CAD build for the part. Positions are in the model's coordinates, mm. Face numbers are marked on the shaded views. A direction names the side the tool comes from. Coordinates: 2 decimals unless noted, no trailing zeros. Loops run counter-clockwise (first coordinate to the right, second up) from the corner with the lowest first, then second, coordinate; pieces in that order, holes last. Notation, with made-up numbers: (71.5, 18.25) -> (128.5, 18.25) arc R32 cw to (128.5, 52.25) -> close; hole circle Ø8 at (50, 28). An arc over 180 degrees is marked (long way). Write item = value, one per line. Start each with the question number.
(1) Band-saw the part on A-A (z = -50). Write the cut outline in (x, y), and give its area (3 significant figures).
(2) Band-saw the part on B-B (y = 37.5). Write the cut outline in (x, z).
(3) Tool access for the marked faces 1 and 2: list every direction of +Z, -Z, +X, -X, +Y, -Y with a clear straight run to the whole face (end or side of a thin tool).
(4) Pull direction Z, two halves, no side cores. Call the marked faces 3, 4 and 5: +Z half, -Z half, draft (parallel to the pull), parting line (faces both ways), or undercut.
(5) Flat gauge pins, fed straight in: P1, Ø1.5, axis at x = 77.5, z = -70, coming from the +Y side; P2, Ø2, axis at x = 15.87, y = 58.37, coming from the +Z side; P3, Ø25, axis at x = 85, y = 65, coming from the -Z side; P4, Ø2, axis at x = 69.2, z = -73.6, coming from the +Y side. Where does each tip first touch, or does it go through?
(6) Band-saw the part on C-C (x = 59). Write the cut outline in (y, z), and give its area (3 significant figures).
(7) Drill centre lines: line 1 (Y direction, x = 30, z = -119.15); line 2 (Y direction, x = 119.15, z = -20); line 3 (Z direction, x = 58, y = 48). Where is each one in solid material? Low to high. Write a range as from..to.
(8) Band-saw the part on D-D (x = 87). Write the cut outline in (y, z), and give its area (3 significant figures).
```python
from build123d import *

# Parameters (mm, degrees)
SKETCH1_W                   = 120
SKETCH1_H                   = 120
BOSS_EXTRUDE1_DEPTH         = 90
SKETCH2_W                   = 116.2
SKETCH2_H                   = 116.2
CUT_EXTRUDE1_DEPTH          = 88
BOSS_EXTRUDE2_DEPTH         = 88
CUT_EXTRUDE2_REACH          = 194.094
SKETCH5_R                   = 4.75
SKETCH5_R_2                 = 15.75
CUT_EXTRUDE3_REACH          = 194.094
SKETCH4_R                   = 3.9
SKETCH4_R_2                 = 15.75
SKETCH4_W                   = 12
SKETCH4_H                   = 10.8
CUT_EXTRUDE4_REACH          = 194.094
SKETCH6_R                   = 4.75
SKETCH6_R_2                 = 3.4
SKETCH6_R_3                 = 9.9
M3_TAPPED_HOLE1_D           = 2.5
M3_TAPPED_HOLE1_CSINK_D     = 3.05
M3_TAPPED_HOLE1_CSINK_ANGLE = 90
M3_TAPPED_HOLE3_D           = 2.5
M3_TAPPED_HOLE3_DEPTH       = 7.5
M3_TAPPED_HOLE3_CSINK_D     = 3.05
M3_TAPPED_HOLE3_CSINK_ANGLE = 90
M3_TAPPED_HOLE3_TIP         = 0.751075774
M3_TAPPED_HOLE4_D           = 2.5
M3_TAPPED_HOLE4_DEPTH       = 7.5
M3_TAPPED_HOLE4_CSINK_D     = 3.05
M3_TAPPED_HOLE4_CSINK_ANGLE = 90
M3_TAPPED_HOLE4_TIP         = 0.751075774


with BuildPart() as part:
    # Sketch1 → Boss-Extrude1 (new body)
    with BuildSketch(Plane(origin=(0, 0, 0), x_dir=(1, 0, 0), z_dir=(0, 1, 0))):
        with Locations((60, 60)):
            Rectangle(SKETCH1_W, SKETCH1_H)
    extrude(amount=BOSS_EXTRUDE1_DEPTH)

    # Sketch2 → Cut-Extrude1 (cut)
    with BuildSketch(Plane(origin=(0, 90, 0), x_dir=(1, 0, 0), z_dir=(0, 1, 0))):
        with Locations((60, 60)):
            Rectangle(SKETCH2_W, SKETCH2_H)
    extrude(amount=-CUT_EXTRUDE1_DEPTH, mode=Mode.SUBTRACT)

    # Sketch3 → Boss-Extrude2 (add)
    with BuildSketch(Plane(origin=(0, 2, 0), x_dir=(1, 0, 0), z_dir=(0, 1, 0))):
        with BuildLine():
            Line((5.9, 118.1), (1.9, 118.1))
            Line((1.9, 118.1), (1.9, 114.1))
            ThreePointArc((1.9, 114.1), (8.728427125, 111.271572875), (5.9, 118.1))
        make_face()
        with BuildLine():
            Line((114.1, 118.1), (118.1, 118.1))
            Line((118.1, 118.1), (118.1, 114.1))
            ThreePointArc((118.1, 114.1), (111.271572875, 111.271572875), (114.1, 118.1))
        make_face()
        with BuildLine():
            Line((118.1, 1.9), (118.1, 5.9))
            ThreePointArc((118.1, 5.9), (111.271572875, 8.728427125), (114.1, 1.9))
            Line((114.1, 1.9), (118.1, 1.9))
        make_face()
        with BuildLine():
            Line((1.9, 1.9), (1.9, 5.9))
            ThreePointArc((1.9, 5.9), (8.728427125, 8.728427125), (5.9, 1.9))
            Line((5.9, 1.9), (1.9, 1.9))
        make_face()
    extrude(amount=BOSS_EXTRUDE2_DEPTH)

    # Sketch5 → Cut-Extrude2 (cut, up to next)
    with BuildSketch(Plane.XY.offset(-120), mode=Mode.PRIVATE) as cut_extrude2_sk1:
        with Locations(Location((30, 75, 0), (0, 0, 180))):
            Circle(SKETCH5_R)
    cut_extrude2_tool1 = extrude(cut_extrude2_sk1.sketch, amount=CUT_EXTRUDE2_REACH, mode=Mode.PRIVATE) & part.part
    # Sketch5 → Cut-Extrude2 (cut, up to next)
    with BuildSketch(Plane.XY.offset(-120), mode=Mode.PRIVATE) as cut_extrude2_sk2:
        with Locations(Location((85, 65, 0), (0, 0, 180))):
            Circle(SKETCH5_R_2)
    cut_extrude2_tool2 = extrude(cut_extrude2_sk2.sketch, amount=CUT_EXTRUDE2_REACH, mode=Mode.PRIVATE) & part.part
    # Sketch5 → Cut-Extrude2 (cut, up to next)
    with BuildSketch(Plane.XY.offset(-120), mode=Mode.PRIVATE) as cut_extrude2_sk3:
        with Locations(Location((30, 60, 0), (0, 0, 180))):
            Circle(SKETCH5_R)
    cut_extrude2_tool3 = extrude(cut_extrude2_sk3.sketch, amount=CUT_EXTRUDE2_REACH, mode=Mode.PRIVATE) & part.part
    # Sketch5 → Cut-Extrude2 (cut, up to next)
    with BuildSketch(Plane.XY.offset(-120), mode=Mode.PRIVATE) as cut_extrude2_sk4:
        with Locations(Location((30, 45, 0), (0, 0, 180))):
            Circle(SKETCH5_R)
    cut_extrude2_tool4 = extrude(cut_extrude2_sk4.sketch, amount=CUT_EXTRUDE2_REACH, mode=Mode.PRIVATE) & part.part
    add(cut_extrude2_tool1.solids().sort_by_distance((30, 75, -120))[0], mode=Mode.SUBTRACT)
    add(cut_extrude2_tool2.solids().sort_by_distance((85, 65, -120))[0], mode=Mode.SUBTRACT)
    add(cut_extrude2_tool3.solids().sort_by_distance((30, 60, -120))[0], mode=Mode.SUBTRACT)
    add(cut_extrude2_tool4.solids().sort_by_distance((30, 45, -120))[0], mode=Mode.SUBTRACT)

    # Sketch4 → Cut-Extrude3 (cut, up to next)
    with BuildSketch(Plane.XY, mode=Mode.PRIVATE) as cut_extrude3_sk1:
        with Locations((60, 78)):
            Circle(SKETCH4_R)
    cut_extrude3_tool1 = extrude(cut_extrude3_sk1.sketch, amount=-CUT_EXTRUDE3_REACH, mode=Mode.PRIVATE) & part.part
    # Sketch4 → Cut-Extrude3 (cut, up to next)
    with BuildSketch(Plane.XY, mode=Mode.PRIVATE) as cut_extrude3_sk2:
        with Locations((33, 58)):
            Circle(SKETCH4_R_2)
    cut_extrude3_tool2 = extrude(cut_extrude3_sk2.sketch, amount=-CUT_EXTRUDE3_REACH, mode=Mode.PRIVATE) & part.part
    # Sketch4 → Cut-Extrude3 (cut, up to next)
    with BuildSketch(Plane.XY, mode=Mode.PRIVATE) as cut_extrude3_sk3:
        with Locations((87, 58)):
            Circle(SKETCH4_R_2)
    cut_extrude3_tool3 = extrude(cut_extrude3_sk3.sketch, amount=-CUT_EXTRUDE3_REACH, mode=Mode.PRIVATE) & part.part
    # Sketch4 → Cut-Extrude3 (cut, up to next)
    with BuildSketch(Plane.XY, mode=Mode.PRIVATE) as cut_extrude3_sk4:
        with Locations((38.7, 12.4)):
            Rectangle(SKETCH4_W, SKETCH4_H)
    cut_extrude3_tool4 = extrude(cut_extrude3_sk4.sketch, amount=-CUT_EXTRUDE3_REACH, mode=Mode.PRIVATE) & part.part
    add(cut_extrude3_tool1.solids().sort_by_distance((60, 78, 0))[0], mode=Mode.SUBTRACT)
    add(cut_extrude3_tool2.solids().sort_by_distance((33, 58, 0))[0], mode=Mode.SUBTRACT)
    add(cut_extrude3_tool3.solids().sort_by_distance((87, 58, 0))[0], mode=Mode.SUBTRACT)
    add(cut_extrude3_tool4.solids().sort_by_distance((38.7, 12.4, 0))[0], mode=Mode.SUBTRACT)

    # Sketch6 → Cut-Extrude4 (cut, up to next)
    with BuildSketch(Plane(origin=(120, 0, 0), x_dir=(0, 0, -1), z_dir=(1, 0, 0)), mode=Mode.PRIVATE) as cut_extrude4_sk1:
        with Locations((95, 55)):
            Circle(SKETCH6_R)
    cut_extrude4_tool1 = extrude(cut_extrude4_sk1.sketch, amount=-CUT_EXTRUDE4_REACH, mode=Mode.PRIVATE) & part.part
    # Sketch6 → Cut-Extrude4 (cut, up to next)
    with BuildSketch(Plane(origin=(120, 0, 0), x_dir=(0, 0, -1), z_dir=(1, 0, 0)), mode=Mode.PRIVATE) as cut_extrude4_sk2:
        with Locations((20, 65)):
            Circle(SKETCH6_R_2)
    cut_extrude4_tool2 = extrude(cut_extrude4_sk2.sketch, amount=-CUT_EXTRUDE4_REACH, mode=Mode.PRIVATE) & part.part
    # Sketch6 → Cut-Extrude4 (cut, up to next)
    with BuildSketch(Plane(origin=(120, 0, 0), x_dir=(0, 0, -1), z_dir=(1, 0, 0)), mode=Mode.PRIVATE) as cut_extrude4_sk3:
        with Locations((50, 65)):
            Circle(SKETCH6_R_2)
    cut_extrude4_tool3 = extrude(cut_extrude4_sk3.sketch, amount=-CUT_EXTRUDE4_REACH, mode=Mode.PRIVATE) & part.part
    # Sketch6 → Cut-Extrude4 (cut, up to next)
    with BuildSketch(Plane(origin=(120, 0, 0), x_dir=(0, 0, -1), z_dir=(1, 0, 0)), mode=Mode.PRIVATE) as cut_extrude4_sk4:
        with Locations((20, 35)):
            Circle(SKETCH6_R_3)
    cut_extrude4_tool4 = extrude(cut_extrude4_sk4.sketch, amount=-CUT_EXTRUDE4_REACH, mode=Mode.PRIVATE) & part.part
    # Sketch6 → Cut-Extrude4 (cut, up to next)
    with BuildSketch(Plane(origin=(120, 0, 0), x_dir=(0, 0, -1), z_dir=(1, 0, 0)), mode=Mode.PRIVATE) as cut_extrude4_sk5:
        with Locations((50, 35)):
            Circle(SKETCH6_R_3)
    cut_extrude4_tool5 = extrude(cut_extrude4_sk5.sketch, amount=-CUT_EXTRUDE4_REACH, mode=Mode.PRIVATE) & part.part
    add(cut_extrude4_tool1.solids().sort_by_distance((120, 55, -95))[0], mode=Mode.SUBTRACT)
    add(cut_extrude4_tool2.solids().sort_by_distance((120, 65, -20))[0], mode=Mode.SUBTRACT)
    add(cut_extrude4_tool3.solids().sort_by_distance((120, 65, -50))[0], mode=Mode.SUBTRACT)
    add(cut_extrude4_tool4.solids().sort_by_distance((120, 35, -20))[0], mode=Mode.SUBTRACT)
    add(cut_extrude4_tool5.solids().sort_by_distance((120, 35, -50))[0], mode=Mode.SUBTRACT)

    # M3 Tapped Hole1 (through all)
    with Locations(Plane(origin=(44.517722268, 2, -162.246849146), x_dir=(1, 0, 0), z_dir=(0, 1, 0))):
        with Locations((-18.417722268, -139.446849146), (-3.217722268, -88.646849146), (24.682277732, -88.646849146), (29.382277732, -140.546849146)):
            CounterSinkHole(M3_TAPPED_HOLE1_D / 2, M3_TAPPED_HOLE1_CSINK_D / 2, counter_sink_angle=M3_TAPPED_HOLE1_CSINK_ANGLE)

    # M3 Tapped Hole3
    with Locations(Plane(origin=(44.517722268, -28.75570348, 0), x_dir=(1, 0, 0), z_dir=(0, 0, 1))):
        with Locations((-28.646696043, 87.124935168), (9.359552373, 87.17416606), (21.605003092, 86.3372409), (59.611251507, 86.386471792)):
            CounterSinkHole(M3_TAPPED_HOLE3_D / 2, M3_TAPPED_HOLE3_CSINK_D / 2, depth=M3_TAPPED_HOLE3_DEPTH, counter_sink_angle=M3_TAPPED_HOLE3_CSINK_ANGLE)
            with Locations((0, 0, -(M3_TAPPED_HOLE3_DEPTH + M3_TAPPED_HOLE3_TIP / 2))):  # 118° drill point
                Cone(0, M3_TAPPED_HOLE3_D / 2, M3_TAPPED_HOLE3_TIP, mode=Mode.SUBTRACT)

    # M3 Tapped Hole4
    with Locations(Plane(origin=(44.517722268, -28.75570348, -120), x_dir=(-1, 0, 0), z_dir=(0, 0, -1))):
        with Locations((-57.611251507, 94.124935168), (-19.605003092, 94.17416606)):
            CounterSinkHole(M3_TAPPED_HOLE4_D / 2, M3_TAPPED_HOLE4_CSINK_D / 2, depth=M3_TAPPED_HOLE4_DEPTH, counter_sink_angle=M3_TAPPED_HOLE4_CSINK_ANGLE)
            with Locations((0, 0, -(M3_TAPPED_HOLE4_DEPTH + M3_TAPPED_HOLE4_TIP / 2))):  # 118° drill point
                Cone(0, M3_TAPPED_HOLE4_D / 2, M3_TAPPED_HOLE4_TIP, mode=Mode.SUBTRACT)


solid = part.part
```
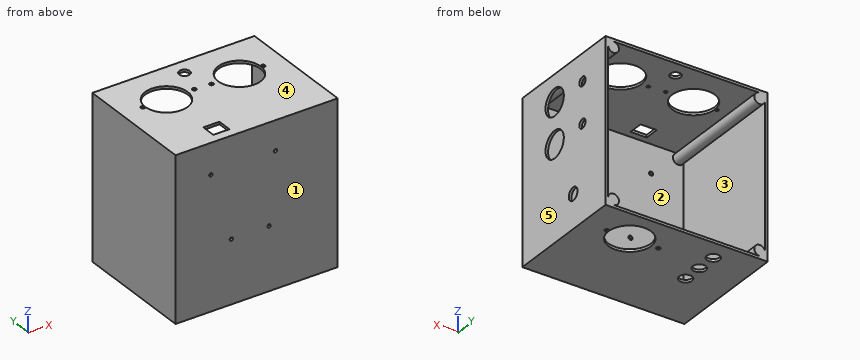
Findings below:
q1.outline = (0, 0) -> (120, 0) -> (120, 25.1) -> (118.1, 25.1) -> (118.1, 2) -> (1.9, 2) -> (1.9, 90) -> (0, 90) -> close; (118.1, 44.9) -> (120, 44.9) -> (120, 61.6) -> (118.1, 61.6) -> close; (118.1, 68.4) -> (120, 68.4) -> (120, 90) -> (118.1, 90) -> close
q1.area = 524 mm²
q2.outline = (0, -120) -> (120, -120) -> (120, -59.58) -> (118.1, -59.58) -> (118.1, -114.1) arc R4 ccw (long way) to (114.1, -118.1) -> (5.9, -118.1) arc R4 ccw (long way) to (1.9, -114.1) -> (1.9, -5.9) arc R4 ccw (long way) to (5.9, -1.9) -> (114.1, -1.9) arc R4 ccw (long way) to (118.1, -5.9) -> (118.1, -10.42) -> (120, -10.42) -> (120, 0) -> (0, 0) -> close; (118.1, -40.42) -> (120, -40.42) -> (120, -29.58) -> (118.1, -29.58) -> close
q3.face_1 = +Z, -Z, +X, -X, -Y
q3.face_2 = +Y
q4.face_3 = undercut
q4.face_4 = +Z half
q4.face_5 = draft
q5.P1 = 2
q5.P2 = -118.1
q5.P3 = -1.9
q5.P4 = through
q6.outline = (0, -120) -> (90, -120) -> (90, -118.1) -> (2, -118.1) -> (2, -1.9) -> (74.23, -1.9) -> (74.23, 0) -> (0, 0) -> close; (81.77, -1.9) -> (90, -1.9) -> (90, 0) -> (81.77, 0) -> close
q6.area = 560 mm²
q7.line_1 = 0..40.25, 49.75..55.25, 64.75..70.25, 79.75..90
q7.line_2 = 0..25.1, 44.9..61.6, 68.4..90
q7.line_3 = -120..-118.1, -1.9..0
q8.outline = (0, -120) -> (49.38, -120) -> (49.38, -118.1) -> (2, -118.1) -> (2, -1.9) -> (42.25, -1.9) -> (42.25, 0) -> (0, 0) -> close; (73.75, -1.9) -> (90, -1.9) -> (90, 0) -> (73.75, 0) -> close; (80.62, -120) -> (90, -120) -> (90, -118.1) -> (80.62, -118.1) -> close
q8.area = 455 mm²
